Geometry: final body of the model. Coordinates: model frame, mm. Face numbers are marked on the shaded views. A direction names the side the tool comes from. Round coordinates to 2 decimals unless told otherwise and drop trailing zeros. Order: outer loops, then holes, each group sorted by start corner. A loop starts at its lowest first (then second) coordinate and runs counter-clockwise, first axis right, second up. Notation, with made-up numbers: (85, -26.5) - (103, -26.5) arc R7 ccw to (103, -21.5) - close; hole circle Ø4 at (-32.5, 72). An arc over 180 degrees is marked (long way). Put each result on its own line as item: value. Start each with the question number.
(1) Pull-direction query (Y, two-part tool) for the marked faces 3, 4, 5 and 6; classes: released by +Y, released by -Y, zero draft, split by the parting line, or undercut.
(2) Section B-B (z = 12). Count the separate pieces of the cut face and the enclosed holes in it, and give its area (3 significant figures).
(3) Section C-C (z = 4). Output: boundary loops of the cut face in (x, y).
(4) Material intervals for L1, parallel to Y at x = 0, z = 14.5; L2, parallel to Y at x = -12.5, z = 13.75; L3, parallel to X at y = -1, z = 14.25, sorted ascending. Write a range as [from, to].
(5) Pin query (flat end, axial travel): P1, Ø10, axis at x = 0, y = 21, coming from the -Z side; P2, Ø8, axis at x = -3, z = 8.5, coming from the -Y side; P3, Ø1, axis at x = -5.5, z = 5.5, coming from the -Y side. Return the tip coordinate at first contact, or that it passes through.
(6) Section A-A (x = 0). Output: boundary loops of the cut face in (y, z), and give its area (4 significant figures).
(7) Access query for the marked faces 1 and 2. Directions: +Z, -Z, +X, -X, +Y, -Y. A direction counts if a zero-diameter tool reaches every point of the face in a straight line with its end or side. Return the directions, or none.
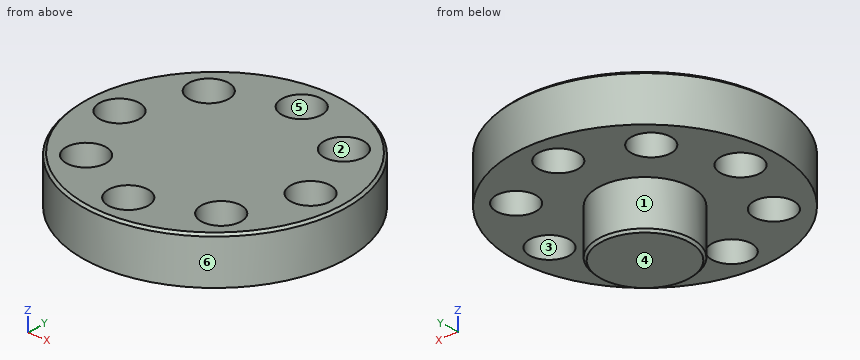
from build123d import *

# Parameters (mm, degrees)
SCHIZZO1_R                   = 10
ESTRUSIONE_ESTRUSIONE1_DEPTH = 10
SCHIZZO2_R                   = 28
ESTRUSIONE_ESTRUSIONE2_DEPTH = 10
SCHIZZO3_R                   = 4.25
TAGLIO_ESTRUSIONE1_DEPTH     = 45.362146026
RIPETIZIONECIRCOLARE1_COUNT  = 8
SMUSSO1_SIZE                 = 0.5
SMUSSO2_SIZE                 = 0.5


with BuildPart() as part:
    # Schizzo1 → Estrusione-Estrusione1 (new body)
    with BuildSketch(Plane.XY):
        Circle(SCHIZZO1_R)
    extrude(amount=ESTRUSIONE_ESTRUSIONE1_DEPTH)

    # Schizzo2 → Estrusione-Estrusione2 (add)
    with BuildSketch(Plane.XY.offset(10)):
        Circle(SCHIZZO2_R)
    extrude(amount=ESTRUSIONE_ESTRUSIONE2_DEPTH)

    # Schizzo3 → Taglio-Estrusione1 (cut, through all)
    with BuildSketch(Plane.XY.offset(20)):
        with Locations((0, 21)):
            Circle(SCHIZZO3_R)
    taglio_estrusione1 = extrude(amount=-TAGLIO_ESTRUSIONE1_DEPTH, mode=Mode.SUBTRACT)

    # RipetizioneCircolare1: Taglio-Estrusione1 ×8 about axis
    ripetizionecircolare1_axis = Axis((0, 0, 0), (0, 0, 1))
    for i in range(1, RIPETIZIONECIRCOLARE1_COUNT):
        add(taglio_estrusione1.rotate(ripetizionecircolare1_axis, i * 360 / RIPETIZIONECIRCOLARE1_COUNT), mode=Mode.SUBTRACT)

    # Smusso1
    smusso1_edges = [part.edges().sort_by_distance(p)[0] for p in [
        (-10, 0, 0),
    ]]
    chamfer(smusso1_edges, length=SMUSSO1_SIZE)

    # Smusso2
    smusso2_edges = [part.edges().sort_by_distance(p)[0] for p in [
        (-28, 0, 20),
    ]]
    chamfer(smusso2_edges, length=SMUSSO2_SIZE)


solid = part.part
Checks:
1. face 3: undercut
1. face 4: zero draft
1. face 5: undercut
1. face 6: split by the parting line
2. separate pieces: 1
2. enclosed holes: 8
2. area: 2,010 mm²
3. outline: circle Ø20 at (0, 0)
4. L1: y = [-28, -25.25], [-16.75, 16.75], [25.25, 28]
4. L2: y = [-25.05, -18.39], [-11.31, 11.31], [18.39, 25.05]
4. L3: x = [-27.98, -25.13], [-16.87, 16.87], [25.13, 27.98]
5. P1: stops at z = 10
5. P2: stops at y = -28
5. P3: stops at y = -8.66
6. outline: (-28, 10) - (-25.25, 10) - (-25.25, 20) - (-27.5, 20) - (-28, 19.5) - close; (-16.75, 10) - (-10, 10) - (-10, 0.5) - (-9.5, 0) - (9.5, 0) - (10, 0.5) - (10, 10) - (16.75, 10) - (16.75, 20) - (-16.75, 20) - close; (25.25, 10) - (28, 10) - (28, 19.5) - (27.5, 20) - (25.25, 20) - close
6. area: 589.5 mm²
7. face 1: -Z
7. face 2: +Z, -Z
